The model under review builds one solid part; all positions refer to its coordinate system, in mm. A direction names the side the tool comes from. Round coordinates to 2 decimals unless told otherwise and drop trailing zeros. Write each loop counter-clockwise with the first axis right and the second up, starting at its lowest first coordinate (ties: lowest second). Pieces come first, ordered by that corner, then holes. Notation, with made-up numbers: (-33, 78.25) -> (-23, 78.25) arc R33 ccw to (-23, 111.25) -> close; hole circle Ø3 at (7, 51.25). An arc over 180 degrees is marked (long way). Use CSV: the item, a comma, the result in double quotes. Start each with the question number.
1) Take a section at B-B, the plane x = -24. Give the boundary of the cut face in (y, z).
2) Take a section at A-A, the plane z = 2.5. Give the boundary of the cut face in (x, y).
3) Take a section at C-C, the plane z = 11.75. Give the boundary of the cut face in (x, y).
4) Machinability: for faces 1 (the face through (1, 1, -1)), 2 (the face through (-1, -49, 6)), which of the approach directions +Z, -Z, +X, -X, +Y, -Y give a long, thin tool a straight path to every point of the face, cutting with its end or side? Answer none if there is none.
5) Wall thickness on probe 1 along Y at (x, z) = (16.5, 3.25); probe 2 along Z at (x, y) = (-38, 3.5): over which ranges is each line inside the solid? List them lowest first. Write a range as [from, to].
6) For pin 1 Ø5 at (x, y) = (20.5, -19.5) entering from +Z, flat-tipped, find the tip position at first contact; note if it passes through.
7) Mouldability with a two-part tool opening along Y and no side actions: class faces 3 (the face through (1, 50, 6)), 4 (the face through (50, -1, 6)), 5 (the face through (1, 1, 0)) as released by +Y, released by -Y, zero draft, split by the parting line, or undercut.
from build123d import *

# Parameters (mm, degrees)
SKETCH1_W           = 100
SKETCH1_H           = 100
SKETCH1_W_2         = 98
SKETCH1_H_2         = 98
BOSS_EXTRUDE1_DEPTH = 13
SKETCH2_W           = 100
SKETCH2_H           = 100
BOSS_EXTRUDE2_DEPTH = 1
SKETCH3_W           = 5
SKETCH3_H           = 5
CUT_EXTRUDE1_DEPTH  = 2


with BuildPart() as part:
    # Sketch1 → Boss-Extrude1 (new body)
    with BuildSketch(Plane.XY):
        Rectangle(SKETCH1_W, SKETCH1_H)
        Rectangle(SKETCH1_W_2, SKETCH1_H_2, mode=Mode.SUBTRACT)
    extrude(amount=BOSS_EXTRUDE1_DEPTH)

    # Sketch2 → Boss-Extrude2 (add)
    with BuildSketch(Plane(origin=(0, 0, 0), x_dir=(-1, 0, 0), z_dir=(0, 0, -1))):
        Rectangle(SKETCH2_W, SKETCH2_H)
    extrude(amount=BOSS_EXTRUDE2_DEPTH)

    # Sketch3 → Cut-Extrude1 (cut)
    with BuildSketch(Plane(origin=(0, 50, 0), x_dir=(1, 0, 0), z_dir=(0, 1, 0))):
        with Locations((5.9, -3.5)):
            Rectangle(SKETCH3_W, SKETCH3_H)
    extrude(amount=-CUT_EXTRUDE1_DEPTH, mode=Mode.SUBTRACT)


solid = part.part
Values found:
1,outline,"(-50, -1) -> (50, -1) -> (50, 13) -> (49, 13) -> (49, 0) -> (-49, 0) -> (-49, 13) -> (-50, 13) -> close"
2,outline,"(-50, -50) -> (50, -50) -> (50, 50) -> (8.4, 50) -> (8.4, 49) -> (49, 49) -> (49, -49) -> (-49, -49) -> (-49, 49) -> (3.4, 49) -> (3.4, 50) -> (-50, 50) -> close"
3,outline,"(-50, -50) -> (50, -50) -> (50, 50) -> (-50, 50) -> close; hole (-49, -49) -> (49, -49) -> (49, 49) -> (-49, 49) -> close"
4,face 1,"-Z, +X, -X, +Y, -Y"
4,face 2,"+Z"
5,probe 1,"[-50, -49], [49, 50]"
5,probe 2,"[-1, 0]"
6,pin 1,"z = 0"
7,face 3,"released by +Y"
7,face 4,"zero draft"
7,face 5,"undercut"
